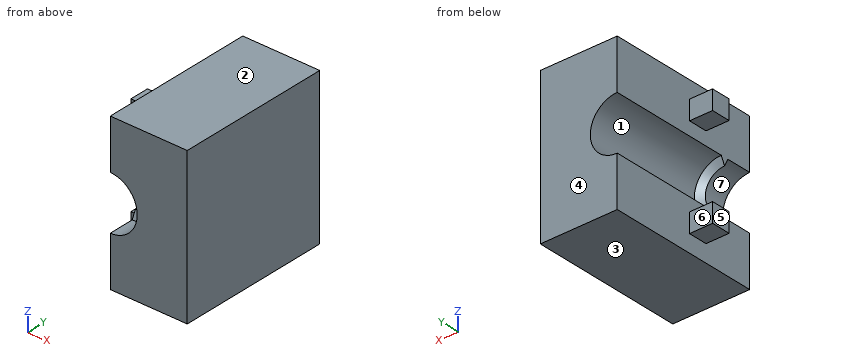
```python
from build123d import *

# Parameters (mm, degrees)
F1_DEPTH  = 10
F3_DEPTH  = 6.7
F5_DEPTH  = 5.7
F8_W      = 2.5
F8_H      = 2.5
F10_DEPTH = 3
F9_W      = 2.5
F9_H      = 2.5
F11_DEPTH = 3
F13_DEPTH = 10
F14_DEPTH = 11


with BuildPart() as f1:
    # F0 (on Front) → F1 (new body)
    with BuildSketch(Plane.XZ):
        with BuildLine():
            ThreePointArc((0, 7), (3.5, 3.5), (0, 0))
            Line((0, 0), (0, -6.5))
            Line((0, -6.5), (10, -6.5))
            Line((10, -6.5), (10, 13.5))
            Line((10, 13.5), (0, 13.5))
            Line((0, 13.5), (0, 7))
        make_face()
    extrude(amount=F1_DEPTH)

    # F2 (on Front) → F3 (join)
    with BuildSketch(Plane.XZ):
        with BuildLine():
            ThreePointArc((0, 6), (2.5, 3.5), (0, 1))
            Line((0, 1), (0, 0))
            ThreePointArc((0, 0), (3.5, 3.5), (0, 7))
            Line((0, 7), (0, 6))
        make_face()
    extrude(amount=F3_DEPTH)

    # F4 (on Front) → F5 (cut)
    with BuildSketch(Plane.XZ):
        with BuildLine():
            Line((0, 1), (0, 0))
            ThreePointArc((0, 0), (3.5, 3.5), (0, 7))
            Line((0, 7), (0, 6))
            ThreePointArc((0, 6), (2.5, 3.5), (0, 1))
        make_face()
    extrude(amount=F5_DEPTH, mode=Mode.SUBTRACT)

    # F6 (on face) → F7 (revolve, cut)
    with BuildSketch(Plane(origin=(0, 0, 0), x_dir=(0, -1, 0), z_dir=(-1, 0, 0))):
        Polygon((6.2, 6), (5.7, 7), (5.7, 6), align=None)
        Polygon((6.7, 7), (6.2, 6), (6.7, 6), align=None)
    revolve(axis=Axis((0, 0, 3.5), (0, 1, 0)), mode=Mode.SUBTRACT)

    # F8 (on face) → F10 (join)
    with BuildSketch(Plane(origin=(0, 0, 0), x_dir=(0, -1, 0), z_dir=(-1, 0, 0))):
        with Locations((2.15, 10)):
            Rectangle(F8_W, F8_H)
    extrude(amount=F10_DEPTH)

    # F9 (on face) → F11 (join)
    with BuildSketch(Plane(origin=(0, 0, 0), x_dir=(0, -1, 0), z_dir=(-1, 0, 0))):
        with Locations((2.15, -3)):
            Rectangle(F9_W, F9_H)
    extrude(amount=F11_DEPTH)

    # F0 (on Front) → F13 (join)
    with BuildSketch(Plane.XZ):
        with BuildLine():
            Line((0, 7), (0, 0))
            ThreePointArc((0, 0), (3.5, 3.5), (0, 7))
        make_face()
        with BuildLine():
            ThreePointArc((0, 7), (3.5, 3.5), (0, 0))
            Line((0, 0), (0, -6.5))
            Line((0, -6.5), (10, -6.5))
            Line((10, -6.5), (10, 13.5))
            Line((10, 13.5), (0, 13.5))
            Line((0, 13.5), (0, 7))
        make_face()
    extrude(amount=-F13_DEPTH)

    # F14 (cut): a face of the model
    f14_faces = [f1.faces().sort_by_distance(p)[0] for p in [
        (1.4854461355, 0, 3.5),
    ]]
    extrude(f14_faces, amount=-F14_DEPTH, mode=Mode.SUBTRACT)


solid = f1.part
```
Read the model definition and answer for the solid it produces. Units are mm, in the model's axes. Face numbers are marked on the shaded views. A direction names the side the tool comes from. Coordinates: 2 decimals unless noted, no trailing zeros. Loops run counter-clockwise (first coordinate to the right, second up) from the corner with the lowest first, then second, coordinate; pieces in that order, holes last. Notation, with made-up numbers: (61.5, 73.25) - (113.5, 73.25) arc R33 ccw to (113.5, 103.25) - close; hole circle Ø2 at (-26.5, 47). An arc over 180 degrees is marked (long way). Answer in a Markdown table with one row per item.
1. Determine the mould class of the marked faces 1, 2, 3 and 4 for opening direction Z: +Z half, -Z half, draft (parallel to the pull), parting line (faces both ways), or undercut.
Conclusion:
| item | result |
|---|---|
| face 1 | undercut |
| face 2 | +Z half |
| face 3 | -Z half |
| face 4 | draft |
2. Find section C-C, the plane y = -2.5. Write down the section's boundary in (x, z).
Conclusion:
| item | result |
|---|---|
| outline | (-3, -4.25) - (0, -4.25) - (0, -6.5) - (10, -6.5) - (10, 13.5) - (0, 13.5) - (0, 11.25) - (-3, 11.25) - (-3, 8.75) - (0, 8.75) - (0, 7) arc R3.5 cw to (0, 0) - (0, -1.75) - (-3, -1.75) - close |
3. Straight lines are drawn through the part: line 1 (X direction, y = -6.25, z = -3.25); line 2 (Z direction, x = 1, y = -3.75); line 3 (Z direction, x = 2.5, y = -1.5). For each, find the intervals that lie inside material, in ascending order.
Conclusion:
| item | result |
|---|---|
| line 1 | x = 0 to 10 |
| line 2 | z = -6.5 to 0.15, 6.85 to 13.5 |
| line 3 | z = -6.5 to 1.05, 5.95 to 13.5 |
4. Find section D-D, the plane z = -0.75. Write down the section's boundary in (x, y), then the cut area to 3 significant figures.
Conclusion:
| item | result |
|---|---|
| outline | (0, -10) - (10, -10) - (10, 10) - (0, 10) - close |
| area | 200 mm² |
5. Find section A-A, the plane z = 3.5. Write down the section's boundary in (x, y), then the cut area to 4 significant figures.
Conclusion:
| item | result |
|---|---|
| outline | (2.5, -6.2) - (3.5, -6.7) - (3.5, -10) - (10, -10) - (10, 10) - (3.5, 10) - (3.5, -5.7) - close |
| area | 130.5 mm² |
6. Given pin 1 (1 mm diameter, centred on y = -0.5, z = -4, fed in from -X); pin 2 (0.8 mm diameter, centred on x = -2, z = 9.5, fed in from +Y); pin 3 (0.8 mm diameter, centred on x = -1, y = -2.5, fed in from -Z); pin 4 (5 mm diameter, centred on y = 3, z = 5, fed in from -X), each flat-ended and moving along its own axis, determine where each tip first touches the part or whether it passes through.
Conclusion:
| item | result |
|---|---|
| pin 1 | stops at x = -3 |
| pin 2 | stops at y = -0.9 |
| pin 3 | stops at z = -4.25 |
| pin 4 | stops at x = 0 |
7. Find section B-B, the plane y = 5.75. Write down the section's boundary in (x, z), then the cut area to 3 significant figures.
Conclusion:
| item | result |
|---|---|
| outline | (0, -6.5) - (10, -6.5) - (10, 13.5) - (0, 13.5) - (0, 7) arc R3.5 cw to (0, 0) - close |
| area | 181 mm² |
8. Which of the six approach directions +Z, -Z, +X, -X, +Y, -Y give full straight-line access (tool end or side, diameter ignored) to the marked faces 5, 6 and 7?
Conclusion:
| item | result |
|---|---|
| face 5 | +Z, -Z, -X, +Y, -Y |
| face 6 | +Z, -Z, -X, +Y |
| face 7 | -X, -Y |
